```python
from build123d import *

# Parameters (mm, degrees)
SKETCH1_R                   = 17.5
SKETCH1_R_2                 = 3
BOSS_EXTRUDE1_DEPTH         = 2
IZIM1_R                     = 4
IZIM1_R_2                   = 3
Y_KSEKLIK_EKSTR_ZYON1_DEPTH = 4
CUT_EXTRUDE1_REACH          = 27.466
SKETCH2_R                   = 1.5


with BuildPart() as part:
    # Sketch1 → Boss-Extrude1 (new body)
    with BuildSketch(Plane(origin=(0, 0, 0), x_dir=(1, 0, 0), z_dir=(0, 1, 0))):
        with Locations(Location((0, 0, 0), (0, 0, 270))):
            Circle(SKETCH1_R)
        with Locations(Location((0, 0, 0), (0, 0, 270))):
            Circle(SKETCH1_R_2, mode=Mode.SUBTRACT)
    extrude(amount=BOSS_EXTRUDE1_DEPTH)

    # Çizim1 → Yükseklik-Ekstrüzyon1 (add)
    with BuildSketch(Plane(origin=(0, 2, 0), x_dir=(1, 0, 0), z_dir=(0, 1, 0))):
        with Locations(Location((0, 0, 0), (0, 0, 270))):
            Circle(IZIM1_R)
        with Locations(Location((0, 0, 0), (0, 0, 270))):
            Circle(IZIM1_R_2, mode=Mode.SUBTRACT)
    extrude(amount=Y_KSEKLIK_EKSTR_ZYON1_DEPTH)

    # Sketch2 → Cut-Extrude1 (cut, up to next)
    with BuildSketch(Plane.XZ, mode=Mode.PRIVATE) as cut_extrude1_sk1:
        with Locations(Location((0, -14, 0), (0, 0, 270))):
            Circle(SKETCH2_R)
    cut_extrude1_tool1 = extrude(cut_extrude1_sk1.sketch, amount=-CUT_EXTRUDE1_REACH, mode=Mode.PRIVATE) & part.part
    add(cut_extrude1_tool1.solids().sort_by_distance((0, 0, -14))[0], mode=Mode.SUBTRACT)


solid = part.part
```
Geometry check sheet. Reference: the model listing, model coordinates, mm. Give positions to 0.01 mm unless a question says otherwise; leave off trailing zeros. Loops run counter-clockwise (first coordinate to the right, second up) from the corner with the lowest first, then second, coordinate; pieces in that order, holes last. Notation, with made-up numbers: M 16.5,47.25 L 23.5,47.25 A34 ccw 23.5,85.25 Z; hole C 4,53.25 d9. An arc over 180 degrees is marked long. Write item = value, one per line. Start each with the question number.
1. Draft check along X on faces 1 (the face through (-3.905, 3.972, -0.867)), 2 (the face through (0.07, 0.99, -12.5)), 3 (the face through (-4, 0, 0)). Enter one of: +X half, -X half, draft (parallel to the pull), parting line (faces both ways), or undercut.
2. Section check B-B, the plane x = 0. Enter the section's corners in (y, z).
3. Section check C-C, the plane y = 3.9. Enter the section's corners in (x, z), plus the area to 3 significant figures.
4. Go/stop test with flat-tipped pins: P1, Ø1, axis at y = 1.5, z = 6.5, coming from the -X side; P2, Ø2, axis at x = 7.5, z = -12.5, coming from the +Y side; P3, Ø1, axis at y = 2, z = -4, coming from the -X side. Record where each tip stops, or that it passes through.
5. Section check D-D, the plane z = -14. Enter the section's corners in (x, y), plus the area to 3 significant figures.
6. Thickness scan on probe 1 along X at (y, z) = (4.5, 0); probe 2 along Y at (x, z) = (6.5, -15); probe 3 along X at (y, z) = (1.5, 0). Record the ranges inside material, lowest first.
7. Section check A-A, the plane z = 0. Enter the section's corners in (x, y).
Values follow:
q1.face_1 = parting line
q1.face_2 = undercut
q1.face_3 = draft
q2.outline = M 0,-17.5 L 2,-17.5 L 2,-15.5 L 0,-15.5 Z; M 0,-12.5 L 2,-12.5 L 2,-4 L 6,-4 L 6,-3 L 0,-3 Z; M 0,3 L 6,3 L 6,4 L 2,4 L 2,17.5 L 0,17.5 Z
q3.outline = C 0,0 d8; hole C 0,0 d6
q3.area = 22.0 mm^2
q4.P1 = -16.44
q4.P2 = 2
q4.P3 = -17.15
q5.outline = M -10.5,0 L -1.5,0 L -1.5,2 L -10.5,2 Z; M 1.5,0 L 10.5,0 L 10.5,2 L 1.5,2 Z
q5.area = 36.0 mm^2
q6.probe_1 = -4 to -3, 3 to 4
q6.probe_2 = 0 to 2
q6.probe_3 = -17.5 to -3, 3 to 17.5
q7.outline = M -17.5,0 L -3,0 L -3,6 L -4,6 L -4,2 L -17.5,2 Z; M 3,0 L 17.5,0 L 17.5,2 L 4,2 L 4,6 L 3,6 Z
